```python
from build123d import *

# Parameters (mm, degrees)
SKETCH1_W                = 30
SKETCH1_H                = 35
BOSS_EXTRUDE1_DEPTH      = 1.6
CUT_EXTRUDE3_DEPTH       = 0.001
M2_CLEARANCE_HOLE1_D     = 2.2
M2_CLEARANCE_HOLE1_DEPTH = 5.2
M2_CLEARANCE_HOLE1_TIP   = 0.660946681
FILLET2_R                = 3


with BuildPart() as part:
    # Sketch1 → Boss-Extrude1 (new body)
    with BuildSketch(Plane(origin=(0, 0, 0), x_dir=(1, 0, 0), z_dir=(0, 1, 0))):
        Rectangle(SKETCH1_W, SKETCH1_H)
    extrude(amount=BOSS_EXTRUDE1_DEPTH)

    # Sketch5 → Cut-Extrude3 (cut)
    with BuildSketch(Plane.XZ):
        with BuildLine():
            Line((7, 17.5), (3, 17.5))
            Line((3, 17.5), (3, 5))
            ThreePointArc((3, 5), (2.267766953, 3.232233047), (0.5, 2.5))
            Line((0.5, 2.5), (-0.5, 2.5))
            ThreePointArc((-0.5, 2.5), (-2.267766953, 3.232233047), (-3, 5))
            Line((-3, 5), (-3, 17.5))
            Line((-3, 17.5), (-7, 17.5))
            Line((-7, 17.5), (-7, -17.5))
            Line((-7, -17.5), (-3, -17.5))
            Line((-3, -17.5), (-3, -7))
            ThreePointArc((-3, -7), (-2.267766953, -5.232233047), (-0.5, -4.5))
            Line((-0.5, -4.5), (0.5, -4.5))
            ThreePointArc((0.5, -4.5), (2.267766953, -5.232233047), (3, -7))
            Line((3, -7), (3, -17.5))
            Line((3, -17.5), (7, -17.5))
            Line((7, -17.5), (7, 17.5))
        make_face()
    extrude(amount=-CUT_EXTRUDE3_DEPTH, mode=Mode.SUBTRACT)

    # M2 Clearance Hole1
    with Locations(Plane(origin=(0, 1.6, 0), x_dir=(1, 0, 0), z_dir=(0, 1, 0))):
        with Locations((-5, 14.5), (-5, -15.4), (5, -15.4), (5, 14.5), (0, 1)):
            Hole(M2_CLEARANCE_HOLE1_D / 2, depth=M2_CLEARANCE_HOLE1_DEPTH)
            with Locations((0, 0, -(M2_CLEARANCE_HOLE1_DEPTH + M2_CLEARANCE_HOLE1_TIP / 2))):  # 118° drill point
                Cone(0, M2_CLEARANCE_HOLE1_D / 2, M2_CLEARANCE_HOLE1_TIP, mode=Mode.SUBTRACT)

    # Fillet2
    fillet2_edges = [part.edges().sort_by_distance(p)[0] for p in [
        (-15, 0.8, -17.5),
        (15, 0.8, -17.5),
        (15, 0.8, 17.5),
        (-15, 0.8, 17.5),
    ]]
    fillet(fillet2_edges, radius=FILLET2_R)


solid = part.part
```
Input: part model. Units: mm. Frame: model coordinates. Coordinates: 2 decimals unless noted, no trailing zeros. Write each loop counter-clockwise with the first axis right and the second up, starting at its lowest first coordinate (ties: lowest second). Pieces come first, ordered by that corner, then holes. Notation, with made-up numbers: (66.5, -31) - (96.5, -31) arc R21 cw to (96.5, -5) - close; hole circle Ø9 at (-19.5, 30.5). An arc over 180 degrees is marked (long way). Put each result on its own line as item: value. Start each with the question number.
1) Cut plane B-B (y = 0.35). Return the cut outline in (x, z), plus the area to 3 significant figures.
2) Cut plane D-D (z = 15.4). State how many separate pieces and enclosed holes the cut face has, plus the area to 3 significant figures.
3) Mould query, pull axis X, two halves, no side actions, for faces 1 (the face through (1, 0.001, 0)), 2 (the face through (5.14, 0.79, 14.31)), 3 (the face through (14.1, 0.81, 16.64)). Classes: pulls with the +X half, pulls with the -X half, needs draft (parallel to the pull), parting line crosses it, or undercut.
4) Cut plane C-C (x = 5). Return the cut outline in (y, z).
5) Ray query, L1, parallel to Z at x = -5, y = 0.8; L2, parallel to X at y = 0.35, z = -14.5; L3, parallel to X at y = 0.6, z = 15. Return the intervals inside material, ascending.
Resolved:
1. outline: (-15, -14.5) arc R3 ccw to (-12, -17.5) - (12, -17.5) arc R3 ccw to (15, -14.5) - (15, 14.5) arc R3 ccw to (12, 17.5) - (-12, 17.5) arc R3 ccw to (-15, 14.5) - close; hole circle Ø2.2 at (-5, -14.5); hole circle Ø2.2 at (-5, 15.4); hole circle Ø2.2 at (0, -1); hole circle Ø2.2 at (5, -14.5); hole circle Ø2.2 at (5, 15.4)
1. area: 1,020 mm2
2. separate pieces: 3
2. enclosed holes: 0
2. area: 40.5 mm2
3. face 1: needs draft
3. face 2: undercut
3. face 3: pulls with the +X half
4. outline: (0, -17.5) - (1.6, -17.5) - (1.6, -15.6) - (0, -15.6) - close; (0, -13.4) - (1.6, -13.4) - (1.6, 14.3) - (0, 14.3) - close; (0, 16.5) - (1.6, 16.5) - (1.6, 17.5) - (0, 17.5) - close
5. L1: z = -17.5 to -15.6, -13.4 to 14.3, 16.5 to 17.5
5. L2: x = -15 to -6.1, -3.9 to 3.9, 6.1 to 15
5. L3: x = -14.96 to -6.02, -3.98 to 3.98, 6.02 to 14.96
